```python
from build123d import *

# Parameters (mm, degrees)
SKETCH1_W               = 116.332
SKETCH1_H               = 177.8
BOSS_EXTRUDE1_DEPTH     = 3
CUT_EXTRUDE1_DEPTH      = 213.496998153
CUT_EXTRUDE1_DEPTH_BACK = 213.496998153
SKETCH3_R               = 2.25
CUT_EXTRUDE2_DEPTH      = 213.496998153
CUT_EXTRUDE2_DEPTH_BACK = 213.496998153
SKETCH4_R               = 2.25
FILLET1_R               = 6.35


with BuildPart() as part:
    # Sketch1 → Boss-Extrude1 (new body)
    with BuildSketch(Plane(origin=(0, 0, 0), x_dir=(1, 0, 0), z_dir=(0, 1, 0))):
        with Locations((58.166, -88.9)):
            Rectangle(SKETCH1_W, SKETCH1_H)
    extrude(amount=BOSS_EXTRUDE1_DEPTH)

    # Sketch3 → Cut-Extrude1 (cut, two sides: drawn at the far end of the back side and taken through both)
    with BuildSketch(Plane(origin=(0, 3, 0), x_dir=(1, 0, 0), z_dir=(0, 1, 0)).offset(-CUT_EXTRUDE1_DEPTH_BACK)):
        with Locations(Location((26.416, -45.72, 0), (0, 0, 270))):
            Circle(SKETCH3_R)
        with Locations(Location((26.416, -58.42, 0), (0, 0, 270))):
            Circle(SKETCH3_R)
        with Locations(Location((89.916, -45.72, 0), (0, 0, 270))):
            Circle(SKETCH3_R)
        with Locations(Location((89.916, -58.42, 0), (0, 0, 270))):
            Circle(SKETCH3_R)
    extrude(amount=CUT_EXTRUDE1_DEPTH + CUT_EXTRUDE1_DEPTH_BACK, mode=Mode.SUBTRACT)

    # Sketch4 → Cut-Extrude2 (cut, two sides: drawn at the far end of the back side and taken through both)
    with BuildSketch(Plane(origin=(0, 3, 0), x_dir=(1, 0, 0), z_dir=(0, 1, 0)).offset(-CUT_EXTRUDE2_DEPTH_BACK)):
        with Locations(Location((40.7035, -31.75, 0), (0, 0, 270))):
            Circle(SKETCH4_R)
        with Locations(Location((75.6285, -31.75, 0), (0, 0, 270))):
            Circle(SKETCH4_R)
        with Locations(Location((40.7035, -146.05, 0), (0, 0, 270))):
            Circle(SKETCH4_R)
        with Locations(Location((75.6285, -146.05, 0), (0, 0, 270))):
            Circle(SKETCH4_R)
    extrude(amount=CUT_EXTRUDE2_DEPTH + CUT_EXTRUDE2_DEPTH_BACK, mode=Mode.SUBTRACT)

    # Fillet1
    fillet1_edges = [part.edges().sort_by_distance(p)[0] for p in [
        (116.332, 1.5, 0),
        (116.332, 1.5, 177.8),
        (0, 1.5, 177.8),
        (0, 1.5, 0),
    ]]
    fillet(fillet1_edges, radius=FILLET1_R)


solid = part.part
```
Model file for the job. Use its own axes, mm. Round coordinates to 2 decimals unless told otherwise and drop trailing zeros. Order: outer loops, then holes, each group sorted by start corner. A loop starts at its lowest first (then second) coordinate and runs counter-clockwise, first axis right, second up. Notation, with made-up numbers: (-16, 5.5) -> (30, 5.5) arc R23 ccw to (30, 30.5) -> close; hole circle Ø2 at (-8, 7). An arc over 180 degrees is marked (long way). Use one line per item in the form item = value.
Item 1: Drill centre lines: line 1 (X direction, y = 1.75, z = 58.42); line 2 (X direction, y = 2.3, z = 31.75); line 3 (Z direction, x = 28, y = 1.45). Where is each one in solid material? Low to high.
Returned:
line_1 = 0 to 24.17, 28.67 to 87.67, 92.17 to 116.33
line_2 = 0 to 38.45, 42.95 to 73.38, 77.88 to 116.33
line_3 = 0 to 44.12, 47.32 to 56.82, 60.02 to 177.8
Item 2: Flat gauge pin, fed straight in: pin 1 Ø4 at (x, z) = (26.416, 58.42) entering from +Y. Where does the tip first touch, or does it go through?
Returned:
pin_1 = through
Item 3: Pull direction X, two halves, no side cores. Call faces 1 (the face through (87.72, 1.48, 57.93)), 2 (the face through (114.42, 1.52, 175.99)), 3 (the face through (1.81, 1.52, 1.91)): released by +X, released by -X, zero draft, split by the parting line, or undercut.
Returned:
face_1 = undercut
face_2 = released by +X
face_3 = released by -X
Item 4: Cut at A-A, the plane z = 31.75. Write the cut outline in (x, y), and give its area (3 significant figures).
Returned:
outline = (0, 0) -> (38.45, 0) -> (38.45, 3) -> (0, 3) -> close; (42.95, 0) -> (73.38, 0) -> (73.38, 3) -> (42.95, 3) -> close; (77.88, 0) -> (116.33, 0) -> (116.33, 3) -> (77.88, 3) -> close
area = 322 mm^2
